from build123d import *

# Parameters (mm, degrees)
F0_R     = 4
F1_DEPTH = 5
F3_DEPTH = 10
F4_R     = 2.25
F5_DEPTH = 5
F6_R     = 2.25
F7_DEPTH = 127.001
F8_R     = 2.25
F9_DEPTH = 5
F10_R    = 10
F11_R    = 15


with BuildPart() as f1:
    # F0 (on Front) → F1 (new body)
    with BuildSketch(Plane.XZ):
        Polygon((75, 77.609202), (-52, 77.609202), (-52, 9.609202), (8, 9.609202), (8, 25.609202), (75, 25.609202), align=None)
        with Locations((-38, 43.609202)):
            Circle(F0_R, mode=Mode.SUBTRACT)
        with Locations((0, 43.609202)):
            Circle(F0_R, mode=Mode.SUBTRACT)
        with Locations((38, 43.609202)):
            Circle(F0_R, mode=Mode.SUBTRACT)
    extrude(amount=F1_DEPTH)

    # F2 (on face) → F3 (join)
    with BuildSketch(Plane(origin=(0, 0, 0), x_dir=(-1, 0, 0), z_dir=(0, 1, 0))):
        Polygon((-75, 77.609202), (-75, 25.609202), (-70, 25.609202), (-70, 72.609202), (47, 72.609202), (47, 14.609202), (-8, 14.609202), (-8, 9.609202), (52, 9.609202), (52, 77.609202), align=None)
    extrude(amount=F3_DEPTH)

    # F4 (on face) → F5 (cut, through all)
    with BuildSketch(Plane(origin=(0, 0, 9.609202), x_dir=(1, 0, 0), z_dir=(0, 0, -1))):
        with Locations((-37, -5)):
            Circle(F4_R)
        with Locations((-2, -5)):
            Circle(F4_R)
    extrude(amount=-F5_DEPTH, mode=Mode.SUBTRACT)

    # F6 (on face) → F7 (cut, through all)
    with BuildSketch(Plane.YZ.offset(75)):
        with Locations((5, 30.609202)):
            Circle(F6_R)
        with Locations((5, 57.609202)):
            Circle(F6_R)
    extrude(amount=-F7_DEPTH, mode=Mode.SUBTRACT)

    # F8 (on face) → F9 (cut, through all)
    with BuildSketch(Plane.XY.offset(77.609202)):
        with Locations((55, 5)):
            Circle(F8_R)
        with Locations((11.5, 5)):
            Circle(F8_R)
        with Locations((-32, 5)):
            Circle(F8_R)
    extrude(amount=-F9_DEPTH, mode=Mode.SUBTRACT)

    # F10
    f10_edges = [f1.edges().sort_by_distance(p)[0] for p in [
        (70, 5, 72.609202),
        (-47, 5, 72.609202),
    ]]
    fillet(f10_edges, radius=F10_R)

    # F11
    f11_edges = [f1.edges().sort_by_distance(p)[0] for p in [
        (75, 2.5, 77.609202),
        (-52, 2.5, 77.609202),
    ]]
    fillet(f11_edges, radius=F11_R)


solid = f1.part
Input: part model. Units: mm. Frame: model coordinates. A direction names the side the tool comes from. Coordinates: 2 decimals unless noted, no trailing zeros. Loops run counter-clockwise (first coordinate to the right, second up) from the corner with the lowest first, then second, coordinate; pieces in that order, holes last.
(1) Set-up query: faces 5 (the face through (-20, 5, 14.609)), 6 (the face through (11, 0, 50)), 7 (the face through (8, -1, 16)), 8 (the face through (-47.49, 2.39, 73.33)), 9 (the face through (-29.854, 5.676, 75.144)). Return all of +Z, -Z, +X, -X, +Y, -Y with unobstructed straight access to the full face (end or side cutting, diameter ignored); none if empty.
(2) Pull-direction query (Y, two-part tool) for faces 1 (the face through (-34.92, 5.86, 12.07)), 2 (the face through (-0.962, 6.996, 12.074)), 3 (the face through (11, -5, 52)), 4 (the face through (-52, 2, 36)); classes: released by +Y, released by -Y, zero draft, split by the parting line, or undercut.
(3) Material intervals for probe 1 along Z at (x, y) = (6, 7.5); probe 2 along Y at (x, z) = (-37, 11.7); probe 3 along X at (y, z) = (0.5, 36), sorted ascending.
(4) First-contact query: pin 1 Ø13 at (x, z) = (-38, 43.61) entering from -Y; pin 2 Ø13 at (x, z) = (0, 43.61) entering from +Y; pin 3 Ø4 at (x, y) = (11.5, 5) entering from +Z; pin 4 Ø4.5 at (x, y) = (50, 2.5) entering from -Z. Flat tips, straight axial feed; report the tip coordinate or a pass-through.
(5) Section A-A on x = 11.5. Return the cut outline in (y, z), then the cut area to 4 significant figures.
(6) Section C-C on z = 41.5. Return the cut outline in (x, y).
(7) Section D-D on y = -3.75. Return the cut outline in (x, z), then the cut area to 3 significant figures.
(8) Section B-B on x = -2. Return the cut outline in (y, z).
Data:
1. face 5: +X, +Y
1. face 6: +Y
1. face 7: -Z, +X, +Y, -Y
1. face 8: +Z, -X, +Y, -Y
1. face 9: +Z
2. face 1: undercut
2. face 2: undercut
2. face 3: released by -Y
2. face 4: zero draft
3. probe 1: z = 9.61 to 14.61, 72.61 to 77.61
3. probe 2: y = -5 to 2.75, 7.25 to 10
3. probe 3: x = -52 to -47, 70 to 75
4. pin 1: stops at y = -5
4. pin 2: stops at y = 0
4. pin 3: passes through
4. pin 4: stops at z = 72.61
5. outline: (-5, 25.61) - (0, 25.61) - (0, 72.61) - (2.75, 72.61) - (2.75, 77.61) - (-5, 77.61) - close; (7.25, 72.61) - (10, 72.61) - (10, 77.61) - (7.25, 77.61) - close
5. area: 287.5 mm2
6. outline: (-52, -5) - (-41.4, -5) - (-41.4, 0) - (-47, 0) - (-47, 10) - (-52, 10) - close; (-34.6, -5) - (-3.4, -5) - (-3.4, 0) - (-34.6, 0) - close; (3.4, -5) - (34.6, -5) - (34.6, 0) - (3.4, 0) - close; (41.4, -5) - (75, -5) - (75, 10) - (70, 10) - (70, 0) - (41.4, 0) - close
7. outline: (-52, 9.61) - (8, 9.61) - (8, 25.61) - (75, 25.61) - (75, 62.61) arc R15 ccw to (60, 77.61) - (-37, 77.61) arc R15 ccw to (-52, 62.61) - close; hole circle Ø8 at (-38, 43.61); hole circle Ø8 at (0, 43.61); hole circle Ø8 at (38, 43.61)
7. area: 7,320 mm2
8. outline: (-5, 9.61) - (2.75, 9.61) - (2.75, 14.61) - (0, 14.61) - (0, 40.15) - (-5, 40.15) - close; (-5, 47.07) - (0, 47.07) - (0, 72.61) - (10, 72.61) - (10, 77.61) - (-5, 77.61) - close; (7.25, 9.61) - (10, 9.61) - (10, 14.61) - (7.25, 14.61) - close
